```python
from build123d import *

# Parameters (mm, degrees)
BOSS_EXTRU_1_DEPTH                           = 18
ESQUISSE2_R                                  = 2
ENL_V_MAT_EXTRU_1_DEPTH                      = 10
TROU_POUR_TARAUDAGE_POUR_TROU_TARAUD_M4_D    = 3.3
TROU_POUR_TARAUDAGE_POUR_TROU_TARAUD_2_D     = 3.3
TROU_POUR_TARAUDAGE_POUR_TROU_TARAUD_2_DEPTH = 7


with BuildPart() as part:
    # Esquisse1 → Boss.-Extru.1 (new body)
    with BuildSketch(Plane(origin=(0, 0, 0), x_dir=(1, 0, 0), z_dir=(0, 1, 0))):
        Polygon((-6, -3.464101615), (0, -6.92820323), (6, -3.464101615), (6, 3.464101615), (0, 6.92820323), (-6, 3.464101615), align=None)
    extrude(amount=BOSS_EXTRU_1_DEPTH)

    # Esquisse2 → Enlèv. mat.-Extru.1 (cut)
    with BuildSketch(Plane(origin=(0, 18, 0), x_dir=(1, 0, 0), z_dir=(0, 1, 0))):
        with Locations(Location((0, 0, 0), (0, 0, 270))):
            Circle(ESQUISSE2_R)
    extrude(amount=-ENL_V_MAT_EXTRU_1_DEPTH, mode=Mode.SUBTRACT)

    # Trou pour taraudage pour trou taraud_ M4 (through all)
    with Locations(Plane(origin=(0, 0, 0), x_dir=(0, 0, -1), z_dir=(0, -1, 0))):
        with Locations((0, 0)):
            Hole(TROU_POUR_TARAUDAGE_POUR_TROU_TARAUD_M4_D / 2)

    # Trou pour taraudage pour trou taraud 2
    with Locations(Plane(origin=(6, 0, 0), x_dir=(0, 0, -1), z_dir=(1, 0, 0))):
        with Locations((0, 12)):
            Hole(TROU_POUR_TARAUDAGE_POUR_TROU_TARAUD_2_D / 2, depth=TROU_POUR_TARAUDAGE_POUR_TROU_TARAUD_2_DEPTH)


solid = part.part
```
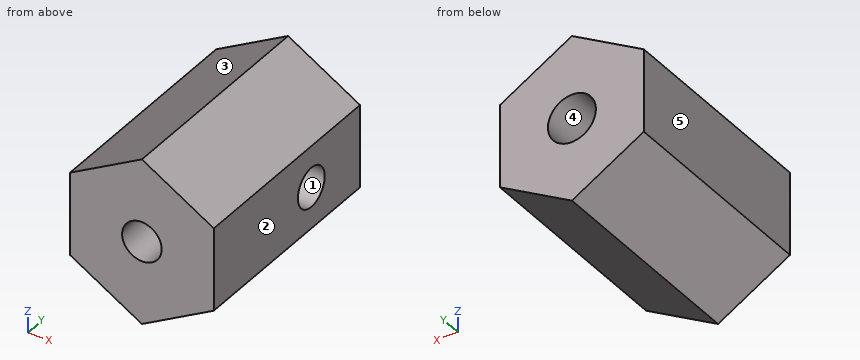
Source: CAD feature listing. Evaluate the final solid. Frame: model axes, mm. Face numbers are marked on the shaded views. A direction names the side the tool comes from. Coordinates: 2 decimals unless noted, no trailing zeros. Loops run counter-clockwise (first coordinate to the right, second up) from the corner with the lowest first, then second, coordinate; pieces in that order, holes last. Notation, with made-up numbers: M 71.25,-0.75 L 81.25,-0.75 A19 cw 81.25,31.25 Z; hole C -7,-15 d6. An arc over 180 degrees is marked long. Put each result on its own line as item: value. Start each with the question number.
1) Cut plane D-D on x = 0.75. Return the cut outline in (y, z).
2) Ray query, L1, parallel to Y at x = 4.3, z = 0; L2, parallel to X at y = 2.5, z = 0; L3, parallel to Z at x = 3.7, y = 12. Return the intervals inside material, ascending. Write a range as from..to.
3) Pull-direction query (Z, two-part tool) for the marked faces 3, 4 and 5; classes: pulls with the +Z half, pulls with the -Z half, needs draft (parallel to the pull), parting line crosses it, or undercut.
4) Reachability of the marked faces 1 and 2 from +Z, -Z, +X, -X, +Y, -Y: full face, straight path, thin tool, end or side. Return the list, or none.
5) Cut plane A-A on z = 0. Return the cut outline in (x, y).
6) Cut plane C-C on y = 12. Return the cut outline in (x, z), then the cut area to 3 significant figures.
7) Contact query for flat-ended pins moving along their axis: pin 1 Ø1 at (x, y) = (-4.5, 6) entering from -Z; pin 2 Ø5 at (x, y) = (-0.5, 5) entering from -Z; pin 3 Ø2 at (x, y) = (-2.5, 14) entering from +Z. Output: stop coordinate, or through.
8) Cut plane B-B on y = 16. Return the cut outline in (x, z), then the cut area to 3 significant figures.
The answers:
1. outline: M 0,-6.5 L 18,-6.5 L 18,-1.85 L 8,-1.85 L 8,-1.47 L 0,-1.47 Z; M 0,1.47 L 8,1.47 L 8,1.85 L 18,1.85 L 18,6.5 L 0,6.5 Z
2. L1: y = 0..10.35, 13.65..18
2. L2: x = -6..-1.65, 1.65..6
2. L3: z = -4.79..-1.65, 1.65..4.79
3. face 3: pulls with the +Z half
3. face 4: undercut
3. face 5: needs draft
4. face 1: +X
4. face 2: +Z, -Z, +X, +Y, -Y
5. outline: M -6,0 L -1.65,0 L -1.65,8 L -2,8 L -2,18 L -6,18 Z; M 1.65,0 L 6,0 L 6,10.35 L 2,10.35 L 2,8 L 1.65,8 Z; M 2,13.65 L 6,13.65 L 6,18 L 2,18 Z
6. outline: M -6,-3.46 L 0,-6.93 L 6,-3.46 L 6,-1.65 L 1.13,-1.65 A2 cw long 1.13,1.65 L 6,1.65 L 6,3.46 L 0,6.93 L -6,3.46 Z
6. area: 98.1 mm²
7. pin 1: stops at z = -4.62
7. pin 2: stops at z = -6.93
7. pin 3: stops at z = 6.06
8. outline: M -6,-3.46 L 0,-6.93 L 6,-3.46 L 6,3.46 L 0,6.93 L -6,3.46 Z; hole C 0,0 d4
8. area: 112 mm²
